Geometry: final body of the model. Coordinates: model frame, mm. Face numbers are marked on the shaded views. Coordinates: 2 decimals unless noted, no trailing zeros. Write each loop counter-clockwise with the first axis right and the second up, starting at its lowest first coordinate (ties: lowest second). Pieces come first, ordered by that corner, then holes. Notation, with made-up numbers: (10.5, 9.5) - (21.5, 9.5) arc R28 ccw to (21.5, 32.5) - close; hole circle Ø8 at (44.5, 32.5). An arc over 180 degrees is marked (long way). Answer as a JSON object with one key per item and string values. Group by question number.
Item 1: Mould query, pull axis Z, two halves, no side actions, for the marked faces 1, 2 and 3. Classes: pulls with the +Z half, pulls with the -Z half, needs draft (parallel to the pull), parting line crosses it, or undercut.
Item 2: First-contact query: pin 1 Ø10 at (y, z) = (22.5, -7) entering from -X; pin 2 Ø3 at (y, z) = (18.5, 11.5) entering from -X; pin 3 Ø1 at (y, z) = (24, -12.5) entering from +X; pin 4 Ø3 at (y, z) = (26.5, 11) entering from +X. Flat tips, straight axial feed; report the tip coordinate or a pass-through.
Item 3: Section D-D on y = 7.5. Return loops of the section in (x, z).
Item 4: Line query: line 1 along X through (y, z) = (16, 0); line 2 along X through (y, z) = (21.5, 5); line 3 along Z through (x, y) = (1, 16). Output: solid intervals per line, ascending. Write a range as from..to.
Item 5: Section C-C on y = 28. Return loops of the section in (x, z).
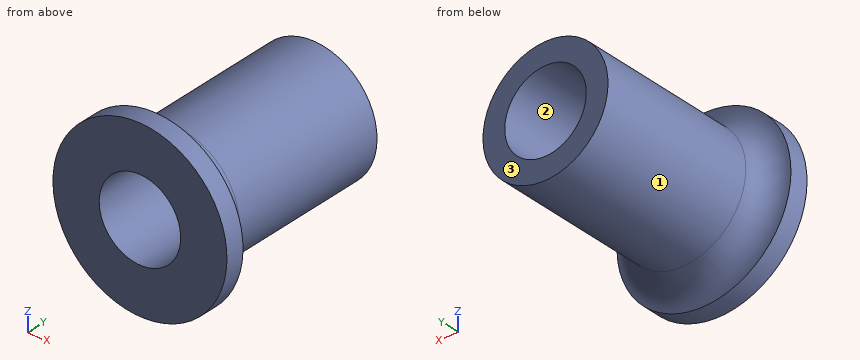
```python
from build123d import *

# Parameters (mm, degrees)
SKETCH_1_R      = 16
SKETCH_1_R_2    = 7.5
EXTRUDE_1_DEPTH = 3.5
SKETCH_2_R      = 11.5
SKETCH_2_R_2    = 7.5
EXTRUDE_2_DEPTH = 34.5
FILLET_3_R      = 4.5


with BuildPart() as part:
    # 草圖1 → 填料-伸長1 (new body)
    with BuildSketch(Plane(origin=(0, 0, 0), x_dir=(1, 0, 0), z_dir=(0, 1, 0))):
        with Locations(Location((0, 0, 0), (0, 0, 270))):
            Circle(SKETCH_1_R)
        with Locations(Location((0, 0, 0), (0, 0, 270))):
            Circle(SKETCH_1_R_2, mode=Mode.SUBTRACT)
    extrude(amount=EXTRUDE_1_DEPTH)

    # 草圖2 → 填料-伸長2 (add)
    with BuildSketch(Plane(origin=(0, 3.5, 0), x_dir=(1, 0, 0), z_dir=(0, 1, 0))):
        with Locations(Location((0, 0, 0), (0, 0, 270))):
            Circle(SKETCH_2_R)
        with Locations(Location((0, 0, 0), (0, 0, 270))):
            Circle(SKETCH_2_R_2, mode=Mode.SUBTRACT)
    extrude(amount=EXTRUDE_2_DEPTH)

    # 圓角3
    fillet_3_edges = [part.edges().sort_by_distance(p)[0] for p in [
        (0, 3.5, -11.5),
    ]]
    fillet(fillet_3_edges, radius=FILLET_3_R - 0.0001)  # a hair under: the kernel refuses the full size


solid = part.part
```
Checks:
{
 "1": {"face 1": "parting line crosses it", "face 2": "undercut", "face 3": "needs draft"},
 "2": {"pin 1": "x = -11.32", "pin 2": "x = -5.68", "pin 3": "through", "pin 4": "x = 6.48"},
 "3": {"outline": "circle Ø23.06 at (0, 0); hole circle Ø15 at (0, 0)"},
 "4": {"line 1": "-11.5..-7.5, 7.5..11.5", "line 2": "-10.36..-5.59, 5.59..10.36", "line 3": "-11.46..-7.43, 7.43..11.46"},
 "5": {"outline": "circle Ø23 at (0, 0); hole circle Ø15 at (0, 0)"}
}
